Could you check a few things on this model? Use its own coordinates, in mm. Give positions to 0.01 mm unless a question says otherwise; leave off trailing zeros. Loops run counter-clockwise (first coordinate to the right, second up) from the corner with the lowest first, then second, coordinate; pieces in that order, holes last. Notation, with made-up numbers: (63, 27) - (84, 27) arc R18 cw to (84, 32) - close; hole circle Ø10 at (49.5, -16). An arc over 180 degrees is marked (long way). Use CSV: the item, a comma, the result in double quotes.
from build123d import *

# Parameters (mm, degrees)
F1_DEPTH = 4.572


with BuildPart() as f1:
    # F0 (on Front) → F1 (new body)
    with BuildSketch(Plane.XZ):
        with BuildLine():
            Line((1.83182, 10.716404), (0, 0))
            Line((0, 0), (2.980503, -2.411659))
            Line((2.980503, -2.411659), (12.981627, -0.742089))
            ThreePointArc((12.981627, -0.742089), (16.633049, 0.943438), (18.917865, 4.253046))
            Line((18.917865, 4.253046), (25.470812, 22.94586))
            Line((25.470812, 22.94586), (5.861357, 15.592153))
            ThreePointArc((5.861357, 15.592153), (3.196287, 13.691717), (1.83182, 10.716404))
        make_face()
        Polygon((2.980503, -2.411659), (0, 0), (-5.900018, -7.051241), (-2.959986, -9.511268), align=None)
    extrude(amount=F1_DEPTH)


solid = f1.part
1) I'm going to push a flat-ended pin straight in: P1, Ø2, axis at y = -3.5, z = -4.5, coming from the +X side. Where does the tip first touch, or does it pass through?
Answer below:
P1,"stops at x = 2.07"
2) I need wall thicknesses on line 1 along Z through (x, y) = (10, -4); line 2 along Z through (x, y) = (11, -1.75); line 3 along X through (y, z) = (-2.15, 9.5). Which ranges of each line are inside material? Lowest first, please.
Answer below:
line 1,"z = -1.24 to 17.14"
line 2,"z = -1.07 to 17.52"
line 3,"x = 1.62 to 20.76"
3) Suppose I cut it at B-B (x = 12.5). Please give me the cut outline in (y, z).
Answer below:
outline,"(-4.57, -0.82) - (0, -0.82) - (0, 18.08) - (-4.57, 18.08) - close"
4) Suppose I cut it at C-C (z = 3.5). Please give me the cut outline in (x, y), plus the area to 3 significant figures.
Answer below:
outline,"(0.6, -4.57) - (18.61, -4.57) - (18.61, 0) - (0.6, 0) - close"
area,"82.3 mm2"
5) Suppose I cut it at A-A (y = -1.05). Please give me the cut outline in (x, z), plus the area to 3 significant figures.
Answer below:
outline,"(-5.9, -7.05) - (-2.96, -9.51) - (2.98, -2.41) - (12.98, -0.74) arc R7.62 ccw to (18.92, 4.25) - (25.47, 22.95) - (5.86, 15.59) arc R6.35 ccw to (1.83, 10.72) - (0, 0) - close"
area,"405 mm2"
